Could you check a few things on this drawing? It's one solid part, dimensions in mm from its lowest x, y, z. A direction names the side the tool comes from. Give positions to 0.01 mm unless a question says otherwise; leave off trailing zeros. Loops run counter-clockwise (first coordinate to the right, second up) from the corner with the lowest first, then second, coordinate; pieces in that order, holes last.
Q1. Suppose I cut it at D-D (x = 3). List the corners of the cut face in (y, z) for me (1 decimal), and give its area (3 significant figures).
Q2. Suppose I cut it at C-C (y = 7.75). List the corners of the cut face in (x, z) for me (1 decimal), and give its area (3 significant figures).
Q3. Suppose I cut it at A-A (z = 6.35). List the corners of the cut face in (x, y) for me.
Q4. I need wall thicknesses on probe 1 along X at (y, z) = (14, 6.35); probe 2 along Z at (x, y) = (19.05, 14.35) (1 decimal); probe 3 along Z at (x, y) = (20, 15.75) (1 decimal). Which ranges of each line are inside material? Lowest first, please.
Q5. I'm going to push flat-ended pins straight in: P1, Ø5, axis at x = 32, y = 7.5, coming from the -Z side (1 decimal); P2, Ø1.5, axis at x = 11, z = 14, coming from the -Y side; P3, Ø4, axis at x = 7.05, z = 30.35, coming from the +Y side; P4, Ø3.5, axis at x = 30.16, y = 8.35, coming from the -Z side. Where does each tip first touch, or does it pass through?
Q6. For the marked faces 1 and 2, which set-ups out of +Z, -Z, +X, -X, +Y, -Y let a thin tool reach every point of the face, with its end or its side?
Q7. Suppose I cut it at B-B (x = 20). List the corners of the cut face in (y, z) for me (1 decimal).
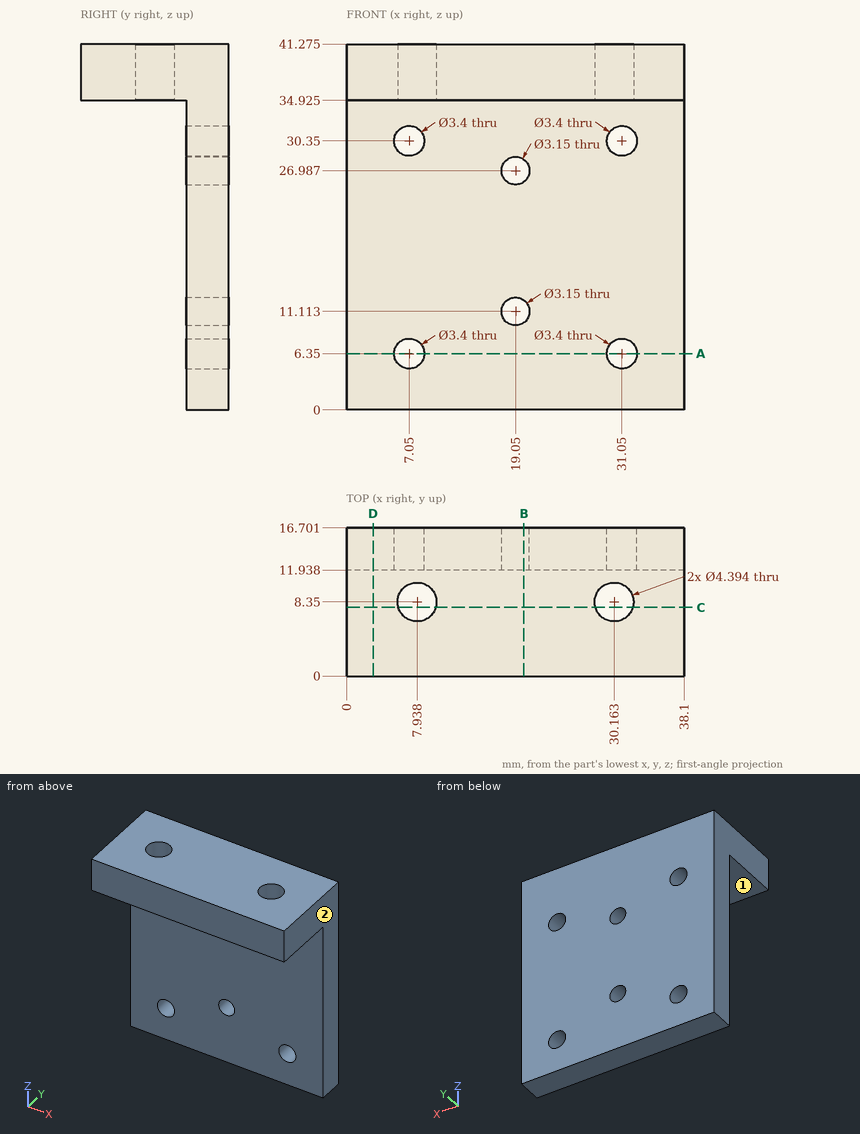
Solutions:
1. outline: (0, 34.9) - (11.9, 34.9) - (11.9, 0) - (16.7, 0) - (16.7, 41.3) - (0, 41.3) - close
1. area: 272 mm2
2. outline: (0, 34.9) - (5.8, 34.9) - (5.8, 41.3) - (0, 41.3) - close; (10.1, 34.9) - (28, 34.9) - (28, 41.3) - (10.1, 41.3) - close; (32.3, 34.9) - (38.1, 34.9) - (38.1, 41.3) - (32.3, 41.3) - close
2. area: 188 mm2
3. outline: (0, 11.94) - (5.35, 11.94) - (5.35, 16.7) - (0, 16.7) - close; (8.75, 11.94) - (29.35, 11.94) - (29.35, 16.7) - (8.75, 16.7) - close; (32.75, 11.94) - (38.1, 11.94) - (38.1, 16.7) - (32.75, 16.7) - close
4. probe 1: x = 0 to 5.35, 8.75 to 29.35, 32.75 to 38.1
4. probe 2: z = 0 to 9.5, 12.7 to 25.4, 28.6 to 41.3
4. probe 3: z = 0 to 9.9, 12.4 to 25.7, 28.2 to 41.3
5. P1: stops at z = 34.9
5. P2: stops at y = 11.94
5. P3: stops at y = 16.7
5. P4: passes through
6. face 1: -Z, +X, -X, -Y
6. face 2: +Z, -Z, +X, +Y, -Y
7. outline: (0, 34.9) - (11.9, 34.9) - (11.9, 28.2) - (16.7, 28.2) - (16.7, 41.3) - (0, 41.3) - close; (11.9, 0) - (16.7, 0) - (16.7, 9.9) - (11.9, 9.9) - close; (11.9, 12.4) - (16.7, 12.4) - (16.7, 25.7) - (11.9, 25.7) - close
